Read the model definition and answer for the solid it produces. Units are mm, in the model's axes. A direction names the side the tool comes from. Give positions to 0.01 mm unless a question says otherwise; leave off trailing zeros. Write each loop counter-clockwise with the first axis right and the second up, starting at its lowest first coordinate (ties: lowest second). Pieces come first, ordered by that corner, then holes.
```python
from build123d import *

# Parameters (mm, degrees)
ISO4762_HEAD_D5P5_H3_SKETCH_R       = 2.75
ISO4762_HEAD_D5P5_H3_DEPTH          = 3
M3_MAJOR_DIAMETER_ENVELOPE_START    = -6
M3_MAJOR_DIAMETER_ENVELOPE_SKETCH_R = 1.5
M3_MAJOR_DIAMETER_ENVELOPE_DEPTH    = 6
HEX_SOCKET_2P5AF_START              = 1.6
HEX_SOCKET_2P5AF_DEPTH              = 1.4


with BuildPart() as part:
    # ISO4762_head_D5p5_h3_Sketch → ISO4762_head_D5p5_h3 (new body)
    with BuildSketch(Plane.XY):
        Circle(ISO4762_HEAD_D5P5_H3_SKETCH_R)
    extrude(amount=ISO4762_HEAD_D5P5_H3_DEPTH)

    # M3_major_diameter_envelope_Sketch → M3_major_diameter_envelope (add)
    with BuildSketch(Plane.XY.offset(M3_MAJOR_DIAMETER_ENVELOPE_START)):
        Circle(M3_MAJOR_DIAMETER_ENVELOPE_SKETCH_R)
    extrude(amount=M3_MAJOR_DIAMETER_ENVELOPE_DEPTH)

    # Hex_socket_2p5AF_Sketch → Hex_socket_2p5AF (cut)
    with BuildSketch(Plane.XY.offset(HEX_SOCKET_2P5AF_START)):
        Polygon((1.443375673, 0), (0.721687836, 1.25), (-0.721687836, 1.25), (-1.443375673, 0), (-0.721687836, -1.25), (0.721687836, -1.25), align=None)
    extrude(amount=HEX_SOCKET_2P5AF_DEPTH, mode=Mode.SUBTRACT)


solid = part.part
```
Item 1: Each of these flat-tipped pins is pushed along its axis until it touches: pin 1 Ø1.5 at (x, y) = (0, 0) entering from +Z; pin 2 Ø0.7 at (x, z) = (-0.5, 2.5) entering from +Y; pin 3 Ø1.5 at (x, z) = (0.5, -5) entering from -Y. Where does it stop, or does it pass through?
Result set:
pin 1: stops at z = 1.6
pin 2: stops at y = 2.75
pin 3: stops at y = -1.5
Item 2: Section C-C (y = 0.5) is taken. Write down the section's boundary in (x, z), and give its area (3 significant figures).
Result set:
outline: (-2.7, 0) - (-1.41, 0) - (-1.41, -6) - (1.41, -6) - (1.41, 0) - (2.7, 0) - (2.7, 3) - (1.15, 3) - (1.15, 1.6) - (-1.15, 1.6) - (-1.15, 3) - (-2.7, 3) - close
area: 30.0 mm2
Item 3: Section A-A (z = 2) is taken. Write down the section's boundary in (x, y), and give its area (3 significant figures).
Result set:
outline: circle Ø5.5 at (0, 0); hole (-1.44, 0) - (-0.72, -1.25) - (0.72, -1.25) - (1.44, 0) - (0.72, 1.25) - (-0.72, 1.25) - close
area: 18.3 mm2
Item 4: Determine the mould class of faces 1 (the flat face through (0, 0, -6)), 2 (the flat face through (1.088, 0.616, 2.29)), 3 (the cylindrical face through (-0.596, -2.685, 1.479)) for opening direction X: pulls with the +X half, pulls with the -X half, needs draft (parallel to the pull), parting line crosses it, or undercut.
Result set:
face 1: needs draft
face 2: undercut
face 3: parting line crosses it
Item 5: Which of the six approach directions +Z, -Z, +X, -X, +Y, -Y give full straight-line access (tool end or side, diameter ignored) to faces 4 (the flat face through (-1.3, -0.6, 3)), 5 (the cylindrical face through (-1.5, 0.07, -3.04)), 6 (the flat face through (0, 1.25, 2))?
Result set:
face 4: +Z, +X, -X, +Y, -Y
face 5: -Z
face 6: +Z
Item 6: Find the intervals of material crossed by line 1 along Y through (x, z) = (-0.4, -4.5); line 2 along Z through (x, y) = (-0.65, 0.65); line 3 along Z through (x, y) = (-1.9, -0.7), in increasing order.
Result set:
line 1: y = -1.45 to 1.45
line 2: z = -6 to 1.6
line 3: z = 0 to 3
Item 7: Section B-B (x = 0) is taken. Write down the section's boundary in (y, z), and give its area (3 significant figures).
Result set:
outline: (-2.75, 0) - (-1.5, 0) - (-1.5, -6) - (1.5, -6) - (1.5, 0) - (2.75, 0) - (2.75, 3) - (1.25, 3) - (1.25, 1.6) - (-1.25, 1.6) - (-1.25, 3) - (-2.75, 3) - close
area: 31.0 mm2
Item 8: Section D-D (z = -3.75) is taken. Write down the section's boundary in (x, y), and give its area (3 significant figures).
Result set:
outline: circle Ø3 at (0, 0)
area: 7.07 mm2
